from build123d import *

# Parameters (mm, degrees)
ESQUISSE1_R        = 13
ESQUISSE1_R_2      = 2.5
BOSS_EXTRU_1_DEPTH = 18


with BuildPart() as part:
    # Esquisse1 → Boss.-Extru.1 (new body)
    with BuildSketch(Plane.XY):
        with BuildLine():
            Line((131.250734203, 99.6547201), (-372.143084144, 25.254923169))
            ThreePointArc((-372.143084144, 25.254923169), (-395.317180347, -1.201804157), (-369.741140617, -25.344367141))
            Line((-369.741140617, -25.344367141), (-0.588044699, -25.344367141))
            ThreePointArc((-0.588044699, -25.344367141), (7.767914285, -24.13176848), (15.262182774, -20.242245906))
            Line((15.262182774, -20.242245906), (146.950608566, 55.788102175))
            ThreePointArc((146.950608566, 55.788102175), (152.209360228, 82.413014403), (131.250734203, 99.6547201))
        make_face()
        with Locations((-370, 0)):
            Circle(ESQUISSE1_R, mode=Mode.SUBTRACT)
        with Locations((127.305734356, 73.5)):
            Circle(ESQUISSE1_R, mode=Mode.SUBTRACT)
        Circle(ESQUISSE1_R, mode=Mode.SUBTRACT)
        with Locations((-223.959522936, 6.655632859)):
            Circle(ESQUISSE1_R_2, mode=Mode.SUBTRACT)
        with Locations((-223.959522936, 26.655632859)):
            Circle(ESQUISSE1_R_2, mode=Mode.SUBTRACT)
    extrude(amount=BOSS_EXTRU_1_DEPTH)


solid = part.part
CAD build for the part. Positions are in the model's coordinates, mm. Give positions to 0.01 mm unless a question says otherwise; leave off trailing zeros. Loops run counter-clockwise (first coordinate to the right, second up) from the corner with the lowest first, then second, coordinate; pieces in that order, holes last. Notation, with made-up numbers: M 64,-8.5 L 74,-8.5 A12 ccw 74,11.5 Z; hole C 3,48.5 d2. An arc over 180 degrees is marked long. One line per question, with ' | ' between items. Start each with the question number.
1. Saw through at D-D on y = 48. Give the cut face in (x, z), plus the area to 3 significant figures.
2. Saw through at C-C on x = 51.5. Give the cut face in (y, z).
3. Flat gauge pins, fed straight in: pin 1 (1 mm diameter, centred on x = -31.5, z = 15.5, fed in from -Y); pin 2 (5 mm diameter, centred on y = 3.5, z = 10, fed in from +X); pin 3 (6 mm diameter, centred on x = -45, z = 15, fed in from +Y); pin 4 (23.5 mm diameter, centred on x = 0, y = 0, fed in from +Z). Where does each tip first touch, or does it go through?
4. Saw through at A-A on y = 73.5. Give the cut face in (x, z), plus the area to 3 significant figures.
5. Saw through at B-B on z = 5.75. Give the cut face in (x, y), plus the area to 3 significant figures.
6. Two-plate mould, pull along X, no slides. Class faces 1 (the face through (-116.922, 62.976, 8.874)), 2 (the face through (-10.316, -7.91, 8.874)), 3 (the face through (-125, 24, 0)): pulls with the +X half, pulls with the -X half, needs draft (parallel to the pull), parting line crosses it, or undercut.
7. Probe L1, parallel to X at y = 3, z = 1.25; L2, parallel to X at y = 8, z = 6.25; L3, parallel to X at y = -5, z = 8. List the from-to ranges inside material, lowest first. Write a range as from..to.
Result sheet:
1) outline: M -218.25,0 L 133.46,0 L 133.46,18 L -218.25,18 Z | area: 6,330 mm^2
2) outline: M 0.68,0 L 87.87,0 L 87.87,18 L 0.68,18 Z
3) pin 1: stops at y = -25.34 | pin 2: stops at x = 60.72 | pin 3: stops at y = 74.05 | pin 4: passes through
4) outline: M -45.71,0 L 114.31,0 L 114.31,18 L -45.71,18 Z; M 140.31,0 L 153.76,0 L 153.76,18 L 140.31,18 Z | area: 3,120 mm^2
5) outline: M -372.14,25.25 A25.35 ccw -369.74,-25.34 L -0.59,-25.34 A25.35 ccw 15.26,-20.24 L 146.95,55.79 A26.45 ccw 131.25,99.65 Z; hole C -370,0 d26; hole C -223.96,6.66 d5; hole C -223.96,26.66 d5; hole C 0,0 d26; hole C 127.31,73.5 d26 | area: 39,800 mm^2
6) face 1: pulls with the -X half | face 2: undercut | face 3: needs draft
7) L1: x = -395.17..-382.65, -357.35..-12.65, 12.65..55.52 | L2: x = -394.05..-380.25, -359.75..-226.07, -221.85..-10.25, 10.25..64.18 | L3: x = -394.85..-382, -358..-12, 12..41.66
